CAD build for the part. Positions are in the model's coordinates, mm. Face numbers are marked on the shaded views. A direction names the side the tool comes from. Coordinates: 2 decimals unless noted, no trailing zeros. Write each loop counter-clockwise with the first axis right and the second up, starting at its lowest first coordinate (ties: lowest second). Pieces come first, ordered by that corner, then holes. Notation, with made-up numbers: (16.25, 52) -> (61.25, 52) arc R21 cw to (61.25, 80) -> close; hole circle Ø4 at (21.25, 10.25). An arc over 180 degrees is marked (long way). Answer as CSV lines item,"result".
```python
from build123d import *

# Parameters (mm, degrees)
SKETCH1_W           = 123.686846594
SKETCH1_H           = 107.02436985
BOSS_EXTRUDE2_DEPTH = 5
SKETCH2_W           = 133.846846594
SKETCH2_H           = 116.939920661
SKETCH2_W_2         = 123.686846594
SKETCH2_H_2         = 107.02436985
BOSS_EXTRUDE4_DEPTH = 20.24
SKETCH4_R           = 2.745
SKETCH4_R_2         = 1.475
BOSS_EXTRUDE5_DEPTH = 12.62
SKETCH5_W           = 12.83643861
SKETCH5_H           = 24.624173529
CUT_EXTRUDE3_DEPTH  = 10


with BuildPart() as part:
    # Sketch1 → Boss-Extrude2 (new body)
    with BuildSketch(Plane(origin=(0, 0, 1258.652497842), x_dir=(-1, 0, 0), z_dir=(0, 0, -1))):
        with Locations((-654.528433331, 841.068613897)):
            Rectangle(SKETCH1_W, SKETCH1_H)
    extrude(amount=-BOSS_EXTRUDE2_DEPTH)

    # Sketch2 → Boss-Extrude4 (add)
    with BuildSketch(Plane(origin=(0, 0, 1258.652497842), x_dir=(-1, 0, 0), z_dir=(0, 0, -1))):
        with Locations((-654.528433331, 841.190838492)):
            Rectangle(SKETCH2_W, SKETCH2_H)
        with Locations((-654.528433331, 841.068613897)):
            Rectangle(SKETCH2_W_2, SKETCH2_H_2, mode=Mode.SUBTRACT)
    extrude(amount=-BOSS_EXTRUDE4_DEPTH)

    # Sketch4 → Boss-Extrude5 (add)
    # profile 1 of 2: a face of its own
    with BuildSketch(Plane.XY.offset(1263.652497842)):
        with Locations(Location((607.327962296, 880.84094357, 0), (0, 0, 180))):
            Circle(SKETCH4_R)
        with Locations((607.327962296, 880.84094357)):
            Circle(SKETCH4_R_2, mode=Mode.SUBTRACT)
    # profile 2 of 2: a face of its own
    with BuildSketch(Plane.XY.offset(1263.652497842)):
        with Locations(Location((702.289411045, 798.927110343, 0), (0, 0, 180))):
            Circle(SKETCH4_R)
        with Locations((702.289411045, 798.927110343)):
            Circle(SKETCH4_R_2, mode=Mode.SUBTRACT)
    extrude(amount=BOSS_EXTRUDE5_DEPTH)

    # Sketch5 → Cut-Extrude3 (cut)
    with BuildSketch(Plane(origin=(721.451856628, 0, 0), x_dir=(0, 0, -1), z_dir=(1, 0, 0))):
        with Locations((-1270.719437851, 837.387376974)):
            Rectangle(SKETCH5_W, SKETCH5_H)
    extrude(amount=-CUT_EXTRUDE3_DEPTH, mode=Mode.SUBTRACT)


solid = part.part
```
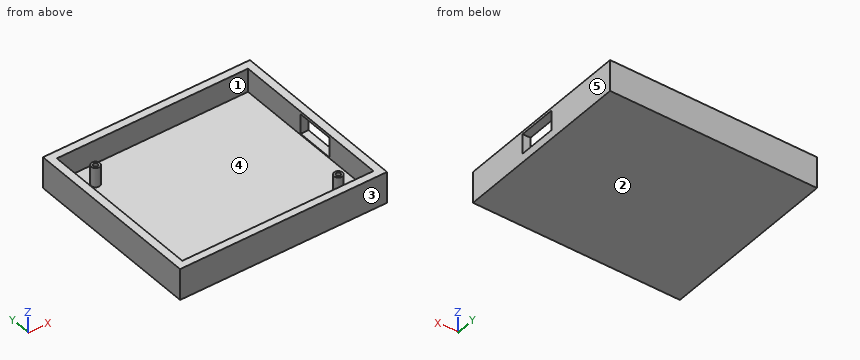
Item 1: Flat gauge pins, fed straight in: pin 1 (4.5 mm diameter, centred on x = 608.5, y = 880.5, fed in from +Z); pin 2 (12 mm diameter, centred on y = 834.5, z = 1269, fed in from +X); pin 3 (1.6 mm diameter, centred on x = 702, y = 799.5, fed in from +Z). Where does each tip first touch, or does it go through?
Answer below:
pin 1,"stops at z = 1276.27"
pin 2,"stops at x = 721.45"
pin 3,"stops at z = 1263.65"
Item 2: Saw through at B-B on z = 1267.5. Give the cut face in (x, y) (3 decimals).
Answer below:
outline,"(587.605, 782.721) -> (721.452, 782.721) -> (721.452, 825.075) -> (716.372, 825.075) -> (716.372, 787.556) -> (592.685, 787.556) -> (592.685, 894.581) -> (716.372, 894.581) -> (716.372, 849.699) -> (721.452, 849.699) -> (721.452, 899.661) -> (587.605, 899.661) -> close; circle Ø5.49 at (607.328, 880.841); circle Ø5.49 at (702.289, 798.927); hole circle Ø2.95 at (607.328, 880.841); hole circle Ø2.95 at (702.289, 798.927)"
Item 3: 3-axis set-ups, long thin cutter, end or side, ignore diameter. For the marked faces 4 and 5: which of +Z, -Z, +X, -X, +Y, -Y reach the whole face in a straight line?
Answer below:
face 4,"+Z"
face 5,"+Z, -Z, +X, +Y, -Y"
Item 4: Wall check: line 1 (Y direction, x = 702, z = 1275.5); line 2 (Y direction, x = 632, z = 1272.25); line 3 (X direction, y = 879, z = 1273.25). Give the ranges that are in metal, low to high. Write a range as from..to.
Answer below:
line 1,"y = 782.72..787.56, 796.2..797.48, 800.37..801.66, 894.58..899.66"
line 2,"y = 782.72..787.56, 894.58..899.66"
line 3,"x = 587.61..592.69, 605.29..609.36, 716.37..721.45"
Item 5: Saw through at D-D on y = 804. Give the cut face in (x, z), and give its area (3 significant figures).
Answer below:
outline,"(587.61, 1258.65) -> (721.45, 1258.65) -> (721.45, 1278.89) -> (716.37, 1278.89) -> (716.37, 1263.65) -> (592.69, 1263.65) -> (592.69, 1278.89) -> (587.61, 1278.89) -> close"
area,"824 mm2"
Item 6: Saw through at C-C on x = 646. Give the cut face in (y, z), and give its area (3 significant figures).
Answer below:
outline,"(782.72, 1258.65) -> (899.66, 1258.65) -> (899.66, 1278.89) -> (894.58, 1278.89) -> (894.58, 1263.65) -> (787.56, 1263.65) -> (787.56, 1278.89) -> (782.72, 1278.89) -> close"
area,"736 mm2"
Item 7: Two-plate mould, pull along Y, no slides. Class the marked faces 1, 2 and 3: pulls with the +Y half, pulls with the -Y half, needs draft (parallel to the pull), parting line crosses it, or undercut.
Answer below:
face 1,"undercut"
face 2,"needs draft"
face 3,"pulls with the -Y half"
Item 8: Saw through at A-A on y = 847. Give the cut face in (x, z).
Answer below:
outline,"(587.61, 1258.65) -> (721.45, 1258.65) -> (721.45, 1264.3) -> (716.37, 1264.3) -> (716.37, 1263.65) -> (592.69, 1263.65) -> (592.69, 1278.89) -> (587.61, 1278.89) -> close; (716.37, 1277.14) -> (721.45, 1277.14) -> (721.45, 1278.89) -> (716.37, 1278.89) -> close"
